```python
from build123d import *

# Parameters (mm, degrees)
BOSS_EXTRUDE1_DEPTH = 10
CHAMFER1_SIZE       = 10
BOSS_EXTRUDE2_START = -10
SKETCH2_R           = 1.4
BOSS_EXTRUDE2_DEPTH = 14.75
CUT_EXTRUDE1_DEPTH  = 5


with BuildPart() as part:
    # Sketch1 → Boss-Extrude1 (new body)
    with BuildSketch(Plane.XY):
        Polygon((0, 0), (28, 0), (38, 10), (-10, 10), align=None)
    extrude(amount=BOSS_EXTRUDE1_DEPTH)

    # Chamfer1
    chamfer1_edges = [part.edges().sort_by_distance(p)[0] for p in [
        (14, 10, 10),
    ]]
    chamfer(chamfer1_edges, length=CHAMFER1_SIZE - 0.0001)  # a hair under: the kernel refuses the full size

    # Sketch2 → Boss-Extrude2 (add)
    with BuildSketch(Plane.XZ.offset(BOSS_EXTRUDE2_START)):
        with Locations(Location((31, 3, 0), (0, 0, 270))):
            Circle(SKETCH2_R)
        with Locations(Location((-3, 3, 0), (0, 0, 90))):
            Circle(SKETCH2_R)
    extrude(amount=BOSS_EXTRUDE2_DEPTH)

    # Sketch4 → Cut-Extrude1 (cut)
    with BuildSketch(Plane(origin=(0, 5, 5), x_dir=(1, 0, 0), z_dir=(0, 0.7071067811865487, 0.7071067811865465))):
        Polygon((-10, 7.071067812), (0, -7.071067812), (28, -7.071067812), (38, 7.071067812), align=None)
    extrude(amount=CUT_EXTRUDE1_DEPTH, mode=Mode.SUBTRACT)


solid = part.part
```
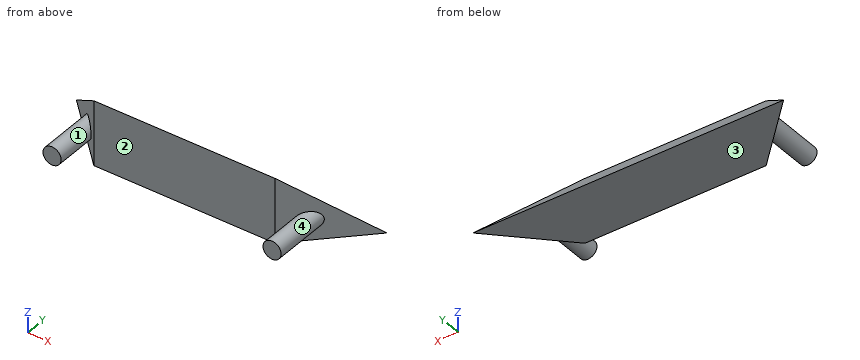
For this review, take the finished solid that the model builds, in its own axes (mm). Face numbers are marked on the shaded views. A direction names the side the tool comes from. Round coordinates to 2 decimals unless told otherwise and drop trailing zeros. Write each loop counter-clockwise with the first axis right and the second up, starting at its lowest first coordinate (ties: lowest second). Pieces come first, ordered by that corner, then holes.
1) Take a section at B-B on x = 31. Give the boundary of the cut face in (y, z).
Answer below:
outline: (-4.75, 1.6) - (3, 1.6) - (3, 0) - (10, 0) - (3, 7) - (3, 4.4) - (-4.75, 4.4) - close
2) Insertion check: pin 1 Ø4 at (y, z) = (0.5, 4) entering from -X; pin 2 Ø1 at (x, y) = (23.5, 1.5) entering from +Z; pin 3 Ø3 at (x, z) = (-4, 5) entering from -Y; pin 4 Ø4 at (x, z) = (9, 7) entering from -Y. Each pin has a flat end and moves straight along its axis. Give the tip position at first contact, or say it passes through.
Answer below:
pin 1: stops at x = -4.4
pin 2: stops at z = 9
pin 3: stops at y = -4.75
pin 4: stops at y = 0
3) For line 1 along X through (y, z) = (-2, 3); line 2 along X through (y, z) = (3, 4); line 3 along Y through (x, z) = (7.5, 6.25), list the stretches that pass through material, from the lowest coordinate up.
Answer below:
line 1: x = -4.4 to -1.6, 29.6 to 32.4
line 2: x = -3.98 to 31.98
line 3: y = 0 to 3.75
4) Take a section at C-C on y = 9.25. Give the boundary of the cut face in (x, z).
Answer below:
outline: (-9.25, 0) - (37.25, 0) - (37.25, 0.75) - (-9.25, 0.75) - close
5) Take a section at A-A on z = 3. Give the boundary of the cut face in (x, y), then the cut area to 3 significant figures.
Answer below:
outline: (-7, 7) - (-4.4, 4.4) - (-4.4, -4.75) - (-1.6, -4.75) - (-1.6, 1.6) - (0, 0) - (28, 0) - (29.6, 1.6) - (29.6, -4.75) - (32.4, -4.75) - (32.4, 4.4) - (35, 7) - close
area: 288 mm2
6) Take a section at D-D on z = 0.5. Give the boundary of the cut face in (x, y).
Answer below:
outline: (-9.5, 9.5) - (0, 0) - (28, 0) - (37.5, 9.5) - close
7) Mouldability with a two-part tool opening along X and no side actions: class the marked faces 3 and 4 as +X half, -X half, draft (parallel to the pull), parting line (faces both ways), or undercut.
Answer below:
face 3: draft
face 4: undercut
8) Machinability: for the marked faces 1 and 2, which of the approach directions +Z, -Z, +X, -X, +Y, -Y give a long, thin tool a straight path to every point of the face, cutting with its end or side? Answer none if there is none.
Answer below:
face 1: -Y
face 2: +Z, -Z, -Y
